from build123d import *

# Parameters (mm, degrees)
SKETCH_2_W          = 340
SKETCH_2_H          = 800
EXTRUDE_1_DEPTH     = 15
SKETCH_3_W          = 310
SKETCH_3_H          = 785
CUT_EXTRUDE_1_DEPTH = 15
SKETCH_8_W          = 310
SKETCH_8_H          = 15
EXTRUDE_3_DEPTH     = 15
CUT_EXTRUDE_5_REACH = 640.949
SKETCH_10_R         = 2
SKETCH_11_R         = 2
CUT_EXTRUDE_6_DEPTH = 819.553864039


with BuildPart() as part:
    # 草图2 → 凸台-拉伸1 (new body)
    with BuildSketch(Plane(origin=(0, 0, 0), x_dir=(1, 0, 0), z_dir=(0, 1, 0))):
        with Locations((2.642487047, -400)):
            Rectangle(SKETCH_2_W, SKETCH_2_H)
    extrude(amount=EXTRUDE_1_DEPTH)

    # 草图3 → 切除-拉伸1 (cut)
    with BuildSketch(Plane(origin=(0, 15, 0), x_dir=(1, 0, 0), z_dir=(0, 1, 0))):
        with Locations((2.642487047, -392.5)):
            Rectangle(SKETCH_3_W, SKETCH_3_H)
    extrude(amount=-CUT_EXTRUDE_1_DEPTH, mode=Mode.SUBTRACT)

    # 草图8 → 凸台-拉伸3 (add)
    with BuildSketch(Plane(origin=(0, 15, 0), x_dir=(1, 0, 0), z_dir=(0, 1, 0))):
        with Locations((2.642487047, -192.5)):
            Rectangle(SKETCH_8_W, SKETCH_8_H)
    extrude(amount=-EXTRUDE_3_DEPTH)

    # 草图10 → 切除-拉伸5 (cut, up to next)
    with BuildSketch(Plane(origin=(0, 0, 185), x_dir=(-1, 0, 0), z_dir=(0, 0, -1)), mode=Mode.PRIVATE) as cut_extrude_5_sk1:
        with Locations((-152.142487047, 7)):
            Circle(SKETCH_10_R)
    cut_extrude_5_tool1 = extrude(cut_extrude_5_sk1.sketch, amount=-CUT_EXTRUDE_5_REACH, mode=Mode.PRIVATE) & part.part
    # 草图10 → 切除-拉伸5 (cut, up to next)
    with BuildSketch(Plane(origin=(0, 0, 185), x_dir=(-1, 0, 0), z_dir=(0, 0, -1)), mode=Mode.PRIVATE) as cut_extrude_5_sk2:
        with Locations((-140.142487047, 7)):
            Circle(SKETCH_10_R)
    cut_extrude_5_tool2 = extrude(cut_extrude_5_sk2.sketch, amount=-CUT_EXTRUDE_5_REACH, mode=Mode.PRIVATE) & part.part
    # 草图10 → 切除-拉伸5 (cut, up to next)
    with BuildSketch(Plane(origin=(0, 0, 185), x_dir=(-1, 0, 0), z_dir=(0, 0, -1)), mode=Mode.PRIVATE) as cut_extrude_5_sk3:
        with Locations((-128.142487047, 7)):
            Circle(SKETCH_10_R)
    cut_extrude_5_tool3 = extrude(cut_extrude_5_sk3.sketch, amount=-CUT_EXTRUDE_5_REACH, mode=Mode.PRIVATE) & part.part
    add(cut_extrude_5_tool1.solids().sort_by_distance((152.142487, 7, 185))[0], mode=Mode.SUBTRACT)
    add(cut_extrude_5_tool2.solids().sort_by_distance((140.142487, 7, 185))[0], mode=Mode.SUBTRACT)
    add(cut_extrude_5_tool3.solids().sort_by_distance((128.142487, 7, 185))[0], mode=Mode.SUBTRACT)

    # 草图11 → 切除-拉伸6 (cut, through all)
    with BuildSketch(Plane(origin=(0, 15, 0), x_dir=(1, 0, 0), z_dir=(0, 1, 0))):
        with Locations(Location((160.142487047, -690, 0), (0, 0, 270))):
            Circle(SKETCH_11_R)
        with Locations(Location((170.142487047, -700, 0), (0, 0, 270))):
            Circle(SKETCH_11_R)
        with Locations(Location((-154.857512953, -690, 0), (0, 0, 270))):
            Circle(SKETCH_11_R)
        with Locations(Location((-164.857512953, -700, 0), (0, 0, 270))):
            Circle(SKETCH_11_R)
    extrude(amount=-CUT_EXTRUDE_6_DEPTH, mode=Mode.SUBTRACT)


solid = part.part
Check sheet for the modelled part. Datum: model origin and axes. Units: mm. A direction names the side the tool comes from. Give positions to 0.01 mm unless a question says otherwise; leave off trailing zeros. Write each loop counter-clockwise with the first axis right and the second up, starting at its lowest first coordinate (ties: lowest second). Pieces come first, ordered by that corner, then holes. Notation, with made-up numbers: (6.25, 74) -> (11.25, 74) arc R21 cw to (11.25, 107) -> close; hole circle Ø8 at (33.25, -5). An arc over 180 degrees is marked (long way). One line per item, written item: value. Start each with the question number.
Item 1: Section check B-B on z = 490.5. Record the cut outline in (x, y), then the cut area to 3 significant figures.
Item 2: Gauge pin test, flat ends, axial feed: pin 1 (8 mm diameter, centred on x = 134, y = 2.5, fed in from -Z); pin 2 (2.5 mm diameter, centred on x = -154.86, z = 690, fed in from -Y). Record the tip position at first contact, or that the pin passes through.
Item 3: Tool access check on faces 4 (the flat face through (2, 15, 191)), 5 (the flat face through (-152.358, 8, 497)), 6 (the flat face through (157.642, 8, 94)). Record the directions out of +Z, -Z, +X, -X, +Y, -Y that give a thin tool (end or side, any length) a straight path to the whole face; none if there is none.
Item 4: Draft check along X on faces 1 (the flat face through (-167.358, 7, 406)), 2 (the flat face through (2, 0, 191)), 3 (the flat face through (0, 8, 785)). Enter one of: +X half, -X half, draft (parallel to the pull), parting line (faces both ways), or undercut.
Item 5: Section check A-A on x = -2. Record the cut outline in (y, z), then the cut area to 3 significant figures.
Item 6: Material ranges on probe 1 along X at (y, z) = (6.25, 700); probe 2 along X at (y, z) = (10.5, 690); probe 3 along Z at (x, y) = (-101, 9), recorded low to high. Write a range as from..to.
Item 7: Section check C-C on y = 11.75. Record the cut outline in (x, z).
Results list:
1. outline: (-167.36, 0) -> (-152.36, 0) -> (-152.36, 15) -> (-167.36, 15) -> close; (157.64, 0) -> (172.64, 0) -> (172.64, 15) -> (157.64, 15) -> close
1. area: 450 mm²
2. pin 1: z = 185
2. pin 2: through
3. face 4: +Z, -Z, +X, -X, +Y
3. face 5: +Y, -Y
3. face 6: -Z, +Y, -Y
4. face 1: -X half
4. face 2: draft
4. face 3: undercut
5. outline: (0, 185) -> (15, 185) -> (15, 200) -> (0, 200) -> close; (0, 785) -> (15, 785) -> (15, 800) -> (0, 800) -> close
5. area: 450 mm²
6. probe 1: -167.36..-166.86, -162.86..-152.36, 157.64..168.14, 172.14..172.64
6. probe 2: -167.36..-156.86, -152.86..-152.36, 157.64..158.14, 162.14..172.64
6. probe 3: 185..200, 785..800
7. outline: (-167.36, 0) -> (-152.36, 0) -> (-152.36, 185) -> (157.64, 185) -> (157.64, 0) -> (172.64, 0) -> (172.64, 800) -> (-167.36, 800) -> close; hole circle Ø4 at (-164.86, 700); hole circle Ø4 at (-154.86, 690); hole (-152.36, 200) -> (157.64, 200) -> (157.64, 785) -> (-152.36, 785) -> close; hole circle Ø4 at (160.14, 690); hole circle Ø4 at (170.14, 700)
